The model under review builds one solid part; all positions refer to its coordinate system, in mm. A direction names the side the tool comes from. Round coordinates to 2 decimals unless told otherwise and drop trailing zeros. Order: outer loops, then holes, each group sorted by start corner. A loop starts at its lowest first (then second) coordinate and runs counter-clockwise, first axis right, second up.
Autodesk Fusion 360 part; units mm, degrees
sketch "Sketch5" plane through (0, 0, 0) normal (0, 0, 1) x (1, 0, 0)
  line L0 (3, 0) -> (61, 0)
  line L1 (64, 3) -> (64, 90)
  line L2 (61, 93) -> (3, 93)
  line L3 (0, 90) -> (0, 3)
  arc A0 (0, 3) -> (3, 0) centre (3, 3) ccw
  arc A1 (3, 93) -> (0, 90) centre (3, 90) ccw
  arc A2 (64, 90) -> (61, 93) centre (61, 90) ccw
  arc A3 (61, 0) -> (64, 3) centre (61, 3) ccw
  point P0 (64, 0)
  point P1 (0, 93)
  dimension "d27" = 64
  dimension "d28" = 93
  dimension "d29" = 3
extrude "Extrude5" add sketch "Sketch5" along normal blind 3
sketch "Sketch6" plane through (0, 0, 0) normal (0, 0, -1) x (1, 0, 0)
  arc A0 (64, -3) -> (61, 0) centre (61, -3) ccw
  line L0 (61, 0) -> (3, 0)
  arc A1 (3, 0) -> (0, -3) centre (3, -3) ccw
  line L1 (0, -3) -> (0, -90)
  arc A2 (0, -90) -> (3, -93) centre (3, -90) ccw
  line L2 (3, -93) -> (61, -93)
  arc A3 (61, -93) -> (64, -90) centre (61, -90) ccw
  line L3 (64, -90) -> (64, -3)
  line L4 (3, -3) -> (61, -3)
  line L5 (61, -3) -> (61, -90)
  line L6 (61, -90) -> (3, -90)
  line L7 (3, -90) -> (3, -3)
  line L8 (3.5, -3) -> (60.5, -3)
  line L9 (60.5, -3) -> (60.5, -6)
  line L10 (60.5, -6) -> (3.5, -6)
  line L11 (3.5, -6) -> (3.5, -3)
  line L12 (3.5, -90) -> (60.5, -90)
  line L13 (60.5, -90) -> (60.5, -87)
  line L14 (60.5, -87) -> (3.5, -87)
  line L15 (3.5, -87) -> (3.5, -90)
  dimension "d32" = 58
  dimension "d33" = 87
  dimension "d34" = 3
  dimension "d35" = 3
  dimension "d36" = 57
  dimension "d37" = 3
  dimension "d38" = 0.5
  dimension "d39" = 57
  dimension "d40" = 3
  dimension "d151" = 0.5
extrude "Extrude6" add sketch "Sketch6" along normal blind 4 contours L4 L8 L9 L10 L11 | L6 L12 L13 L14 L15
sketch "Sketch8" plane through (0, 0, 0) normal (0, 0, -1) x (1, 0, 0)
  line L0 (3.5, -6) -> (3.5, -3)
  line L1 (3.5, -3) -> (60.5, -3)
  line L2 (60.5, -3) -> (60.5, -6)
  line L3 (60.5, -6) -> (3.5, -6)
  line L4 (3.5, -87) -> (60.5, -87)
  line L5 (60.5, -87) -> (60.5, -90)
  line L6 (60.5, -90) -> (3.5, -90)
  line L7 (3.5, -90) -> (3.5, -87)
  arc A0 (64, -3) -> (61, 0) centre (61, -3) ccw
  line L8 (61, 0) -> (3, 0)
  arc A1 (3, 0) -> (0, -3) centre (3, -3) ccw
  line L9 (0, -3) -> (0, -90)
  arc A2 (0, -90) -> (3, -93) centre (3, -90) ccw
  line L10 (3, -93) -> (61, -93)
  arc A3 (61, -93) -> (64, -90) centre (61, -90) ccw
  line L11 (64, -90) -> (64, -3)
  circle A4 centre (15.94, -61.99) radius 1.27
  circle A5 centre (15.94, -78.61) radius 1.27
  circle A6 centre (50.9, -78.61) radius 1.27
  circle A7 centre (50.9, -61.99) radius 1.27
  line L12 (64, -81) -> (0, -81)
  line L13 (0, -81) -> (0, -59.6)
  line L14 (0, -59.6) -> (64, -59.6)
  line L15 (64, -59.6) -> (64, -81)
  dimension "d52" = 2.54
  dimension "d55" = 2.54
  dimension "d58" = 2.54
  dimension "d61" = 2.54
  dimension "d85" = 64
  dimension "d86" = 21.4
  dimension "d87" = 6
  dimension "d92" = 2.39
  dimension "d93" = 2.39
  dimension "d96" = 2.39
  dimension "d97" = 15.94
  dimension "d98" = 2.39
  dimension "d99" = 15.94
  dimension "d100" = 50.9
  dimension "d101" = 50.9
extrude "Extrude8" cut sketch "Sketch8" against normal blind 3 contours A4 | A5 | A6 | A7
sketch "Sketch9" plane through (0, 0, 0) normal (0, 0, -1) x (1, 0, 0)
  circle A0 centre (50.9, -61.99) radius 1.27
  circle A1 centre (50.9, -78.61) radius 1.27
  circle A2 centre (15.94, -61.99) radius 1.27
  circle A3 centre (15.94, -78.61) radius 1.27
  line L0 (3.5, -6) -> (3.5, -3)
  line L1 (3.5, -3) -> (60.5, -3)
  line L2 (60.5, -3) -> (60.5, -6)
  line L3 (60.5, -6) -> (3.5, -6)
  line L4 (3.5, -87) -> (60.5, -87)
  line L5 (60.5, -87) -> (60.5, -90)
  line L6 (60.5, -90) -> (3.5, -90)
  line L7 (3.5, -90) -> (3.5, -87)
  arc A4 (64, -3) -> (61, 0) centre (61, -3) ccw
  line L8 (61, 0) -> (3, 0)
  arc A5 (3, 0) -> (0, -3) centre (3, -3) ccw
  line L9 (0, -3) -> (0, -90)
  arc A6 (0, -90) -> (3, -93) centre (3, -90) ccw
  line L10 (3, -93) -> (61, -93)
  arc A7 (61, -93) -> (64, -90) centre (61, -90) ccw
  line L11 (64, -90) -> (64, -3)
  circle A8 centre (8, -40) radius 1.27
  circle A9 centre (8, -55) radius 1.27
  circle A10 centre (15.5, -40) radius 1.27
  circle A11 centre (15.5, -55) radius 1.27
  line L12 (9, -42) -> (14, -42)
  line L13 (14, -42) -> (14, -53)
  line L14 (14, -53) -> (9, -53)
  line L15 (9, -53) -> (9, -42)
  line L16 (14, -53) -> (22.5, -53)
  line L17 (22.5, -53) -> (22.5, -42)
  line L18 (22.5, -42) -> (14, -42)
  line L19 (14, -42) -> (14, -53)
  dimension "d70" = 2.54
  dimension "d73" = 2.54
  dimension "d76" = 2.54
  dimension "d79" = 2.54
extrude "Extrude9" cut sketch "Sketch9" against normal blind 3 contours A8 | A9 | A10 | A11 | L12 L13 L14 L15 L19
fillet "Fillet5" radius 1.5 4 edges at (32, 3, -4) (32, 6, -4) (32, 87, -4) (32, 90, -4)
sketch "Sketch11" plane through (0, 0, 3) normal (0, 0, 1) x (-1, 0, 0)
  circle A0 centre (-50.9, -61.99) radius 1.27
  circle A1 centre (-50.9, -78.61) radius 1.27
  circle A2 centre (-15.94, -61.99) radius 1.27
  circle A3 centre (-15.94, -78.61) radius 1.27
  arc A4 (-61, 0) -> (-64, -3) centre (-61, -3) ccw
  line L0 (-64, -3) -> (-64, -90)
  arc A5 (-64, -90) -> (-61, -93) centre (-61, -90) ccw
  line L1 (-61, -93) -> (-3, -93)
  arc A6 (-3, -93) -> (0, -90) centre (-3, -90) ccw
  line L2 (0, -90) -> (0, -3)
  arc A7 (0, -3) -> (-3, 0) centre (-3, -3) ccw
  line L3 (-3, 0) -> (-61, 0)
  line L4 (-14, -53) -> (-14, -42)
  line L5 (-14, -42) -> (-9, -42)
  line L6 (-9, -42) -> (-9, -53)
  line L7 (-9, -53) -> (-14, -53)
  circle A8 centre (-15.5, -40) radius 1.27
  circle A9 centre (-8, -55) radius 1.27
  circle A10 centre (-8, -40) radius 1.27
  circle A11 centre (-15.5, -55) radius 1.27
sketch "Sketch12" plane through (0, 0, 3) normal (0, 0, 1) x (-1, 0, 0)
  line L0 (-6.497, -13.503) -> (-6.497, -37.303)
  line L1 (-6.497, -37.303) -> (-31.497, -37.303)
  line L2 (-31.497, -37.303) -> (-31.497, -13.503)
  line L3 (-31.497, -13.503) -> (-6.497, -13.503)
  circle A0 centre (-8.497, -15.503) radius 1.1
  circle A1 centre (-29.297, -15.503) radius 1.1
  circle A2 centre (-8.497, -28.003) radius 1.1
  circle A3 centre (-29.297, -28.003) radius 1.1
  line L4 (-12.997, -19.403) -> (-12.997, -31.403)
  line L5 (-12.997, -31.403) -> (-24.997, -31.403)
  line L6 (-24.997, -31.403) -> (-24.997, -19.403)
  line L7 (-24.997, -19.403) -> (-12.997, -19.403)
  line L8 (-8, -41.3) -> (-15.5, -41.3)
  line L9 (-15.5, -41.3) -> (-15.5, -38.7)
  line L10 (-15.5, -38.7) -> (-8, -38.7)
  line L11 (-8, -38.7) -> (-8, -41.3)
  line L12 (-15.5, -56.3) -> (-8, -56.3)
  line L13 (-8, -56.3) -> (-8, -53.7)
  line L14 (-8, -53.7) -> (-15.5, -53.7)
  line L15 (-15.5, -53.7) -> (-15.5, -56.3)
  line L16 (-54, -76) -> (-45, -76)
  line L17 (-45, -76) -> (-45, -65)
  line L18 (-45, -65) -> (-54, -65)
  line L19 (-54, -65) -> (-54, -76)
  line L20 (-7.3994, -28.077) -> (-9.5994, -28.077)
  line L21 (-9.5994, -28.077) -> (-9.5994, -13.503)
  line L22 (-9.5994, -13.503) -> (-7.3994, -13.503)
  line L23 (-7.3994, -13.503) -> (-7.3994, -28.077)
  line L24 (-28.1994, -28.077) -> (-30.3994, -28.077)
  line L25 (-30.3994, -28.077) -> (-30.3994, -13.503)
  line L26 (-30.3994, -13.503) -> (-28.1994, -13.503)
  line L27 (-28.1994, -13.503) -> (-28.1994, -28.077)
  arc A4 (-7.3994, -13.503) -> (-9.5994, -13.503) centre (-8.4994, -13.503) ccw
  arc A5 (-28.1994, -13.503) -> (-30.3994, -13.503) centre (-29.2994, -13.503) ccw
  dimension "d106" = 23.8
  dimension "d107" = 25
  dimension "d108" = 2.2
  dimension "d109" = 2
  dimension "d110" = 2
  dimension "d111" = 2.2
  dimension "d112" = 2
  dimension "d113" = 2.2
  dimension "d114" = 2.2
  dimension "d115" = 2
  dimension "d116" = 14.5
  dimension "d117" = 2.2
  dimension "d118" = 2.2
  dimension "d119" = 14.5
  dimension "d120" = 12
  dimension "d121" = 12
  dimension "d122" = 6.5
  dimension "d123" = 5.9
  dimension "d143" = 2.2
  dimension "d144" = 14.574
  dimension "d145" = 2.2
  dimension "d146" = 14.574
extrude "Extrude10" cut sketch "Sketch12" against normal blind 3 contours L3 A0 A2 L20 L21 L22 L23 | L3 L22 A4 | A0 L23 | A0 L23 | L3 A1 A3 L24 L25 L26 L27 | L3 L26 A5 | A1 L27 | A1 L27 | A2 L20 | A2 L20 L23 | A2 L23 | A3 L24 | A3 L24 L27 | A3 L27 | L4 L5 L6 L7
sketch "Sketch13" plane through (0, 0, 3) normal (0, 0, 1) x (-1, 0, 0)
  line L0 (-29, -55.0268) -> (-31.8, -55.0268)
  line L1 (-31.8, -55.0268) -> (-31.8, -39.0268)
  line L2 (-31.8, -39.0268) -> (-29, -39.0268)
  line L3 (-29, -39.0268) -> (-29, -55.0268)
  arc A0 (-31.8, -55.0268) -> (-29, -55.0268) centre (-30.4, -55.0268) ccw
  arc A1 (-29, -39.0268) -> (-31.8, -39.0268) centre (-30.4, -39.0268) ccw
  line L4 (-33.8, -55) -> (-48.8, -55)
  line L5 (-48.8, -55) -> (-48.8, -39)
  line L6 (-48.8, -39) -> (-33.8, -39)
  line L7 (-33.8, -39) -> (-33.8, -55)
  line L8 (-14, -42) -> (-14, -53)
  line L9 (-29, -50.0268) -> (-31.8, -50.0268)
  line L10 (-31.8, -50.0268) -> (-31.8, -44.0268)
  line L11 (-31.8, -44.0268) -> (-29, -44.0268)
  line L12 (-29, -44.0268) -> (-29, -50.0268)
  line L13 (-29, -52.0268) -> (-31.8, -52.0268)
  line L14 (-31.8, -52.0268) -> (-31.8, -42.0268)
  line L15 (-31.8, -42.0268) -> (-29, -42.0268)
  line L16 (-29, -42.0268) -> (-29, -52.0268)
  line L17 (-31.8, -50.0268) -> (-33.8, -50.0268)
  line L18 (-33.8, -50.0268) -> (-33.8, -44.0268)
  line L19 (-33.8, -44.0268) -> (-31.8, -44.0268)
  line L20 (-31.8, -44.0268) -> (-31.8, -50.0268)
  line L21 (-14, -53) -> (-21.5354, -53)
  line L22 (-21.5354, -53) -> (-21.5354, -42)
  line L23 (-21.5354, -42) -> (-14, -42)
  line L24 (-14, -42) -> (-14, -53)
  dimension "d126" = 2.8
  dimension "d127" = 16
  dimension "d128" = 15
  dimension "d129" = 16
  dimension "d130" = 2
  dimension "d133" = 15
  dimension "d134" = 6
  dimension "d135" = 5
  dimension "d136" = 2.8
  dimension "d137" = 10
  dimension "d138" = 3
extrude "Extrude12" cut sketch "Sketch13" against normal blind 3 contours L0 A0 | L0 L1 L3 L13 | L1 L3 L9 L10 L11 L12 L14 L16 L20 | L1 L7 L10 L14 L17 L18 L19 L20 | L4 L5 L6 L7 L18 | L1 L2 L3 L15 | L2 A1
extrude "Extrude13" cut sketch "Sketch12" against normal blind 3 contours L8 L9 L10 L11 | L12 L13 L14 L15 | L16 L17 L18 L19
extrude "Extrude14" cut sketch "Sketch13" against normal blind 3 contours L8 L21 L22 L23 L24
sketch "Sketch14" plane through (0, 0, 3) normal (0, 0, 1) x (-1, 0, 0)
  line L0 (-18, -38.7) -> (-26.5, -38.7)
  line L1 (-26.5, -38.7) -> (-26.5, -56.5)
  line L2 (-26.5, -56.5) -> (-18, -56.5)
  line L3 (-18, -56.5) -> (-18, -38.7)
extrude "Extrude15" cut sketch "Sketch14" against normal blind 3
(1) Insertion check: pin 1 (5 mm diameter, centred on x = 13, y = 73.5, fed in from -Z); pin 2 (0.9 mm diameter, centred on y = 5, z = -2.5, fed in from +X); pin 3 (2 mm diameter, centred on x = 15.5, y = 21.5, fed in from +Z); pin 4 (1.3 mm diameter, centred on x = 44.5, z = -1, fed in from +Y). Each pin has a flat end and moves straight along its axis. Give the tip position at first contact, or say it passes through.
Data:
pin 1: stops at z = 0
pin 2: stops at x = 60.5
pin 3: passes through
pin 4: stops at y = 90
(2) Draft analysis for pull direction Y (two halves, no side actions). For faces 1 (the cylindrical face through (8.475, 12.403, 1.521)), 2 (the cylindrical face through (0.86, 92.1, 1.48)), 3 (the flat face through (32, 3, -1)), state which applies: pulls with the +Y half, pulls with the -Y half, needs draft (parallel to the pull), parting line crosses it, or undercut.
Data:
face 1: undercut
face 2: pulls with the +Y half
face 3: pulls with the -Y half
(3) Consider section A-A (y = 40). Write out the cut boundary in (x, z), and give its area (3 significant figures).
Data:
outline: (0, 0) - (6.73, 0) - (6.73, 3) - (0, 3) - close; (16.77, 0) - (18, 0) - (18, 3) - (16.77, 3) - close; (26.5, 0) - (29, 0) - (29, 3) - (26.5, 3) - close; (31.8, 0) - (33.8, 0) - (33.8, 3) - (31.8, 3) - close; (48.8, 0) - (64, 0) - (64, 3) - (48.8, 3) - close
area: 83.0 mm2
(4) Consider section C-C (y = 61.99). Write out the cut boundary in (x, z).
Data:
outline: (0, 0) - (14.67, 0) - (14.67, 3) - (0, 3) - close; (17.21, 0) - (49.63, 0) - (49.63, 3) - (17.21, 3) - close; (52.17, 0) - (64, 0) - (64, 3) - (52.17, 3) - close
(5) For faces 4 (the flat face through (60.5, 89, -2)), 5 (the flat face through (32, 90, -1)), 6 (the flat face through (28.199, 22, 2)), list the 3-axis set-ups (+Z, -Z, +X, -X, +Y, -Y) from which the entire face can be reached by the end or side of a thin tool; tool diameter is ignored.
Data:
face 4: -Z, +X, +Y, -Y
face 5: -Z, +X, -X, +Y
face 6: +Z, -Z
(6) Consider section D-D (z = -1.25). Write out the cut boundary in (x, y), and give its area (3 significant figures).
Data:
outline: (3.5, 3) - (60.5, 3) - (60.5, 6) - (3.5, 6) - close; (3.5, 87) - (60.5, 87) - (60.5, 90) - (3.5, 90) - close
area: 342 mm2
(7) To check wall thickness, follow probe 1 along Y at (x, z) = (50.9, 1.15); probe 2 along Y at (x, z) = (46.5, 1.5); probe 3 along X at (y, z) = (78.61, 1.95). State the ranges of each line that lie inside material, in increasing order.
Data:
probe 1: y = 0 to 60.72, 63.26 to 65, 76 to 77.34, 79.88 to 93
probe 2: y = 0 to 39, 55 to 65, 76 to 93
probe 3: x = 0 to 14.67, 17.21 to 49.63, 52.17 to 64
